Read the model definition and answer for the solid it produces. Units are mm, in the model's axes. Face numbers are marked on the shaded views. A direction names the side the tool comes from. Coordinates: 2 decimals unless noted, no trailing zeros. Loops run counter-clockwise (first coordinate to the right, second up) from the corner with the lowest first, then second, coordinate; pieces in that order, holes last. Notation, with made-up numbers: (9.25, -30.75) -> (23.25, -30.75) arc R15 ccw to (23.25, -5.75) -> close; hole circle Ø11 at (2, 54). An arc over 180 degrees is marked (long way). Answer in a Markdown table with one row per item.
```python
from build123d import *

# Parameters (mm, degrees)
BASE_EXTRUDE_DEPTH = 12.7
LPATTERN1_COUNT    = 2
LPATTERN1_PITCH    = 41.27246


with BuildPart() as part:
    # Sketch1 → Base-Extrude (new, symmetric)
    with BuildSketch(Plane.XY):
        with BuildLine():
            Line((-20.6375, 36.5125), (-20.6375, 2.6924))
            ThreePointArc((-20.6375, 2.6924), (-19.848914298, 0.788585702), (-17.9451, 0))
            Line((-17.9451, 0), (17.9451, 0))
            ThreePointArc((17.9451, 0), (19.848914298, 0.788585702), (20.6375, 2.6924))
            Line((20.6375, 2.6924), (20.6375, 36.5125))
            ThreePointArc((20.6375, 36.5125), (15.875, 41.275), (11.1125, 36.5125))
            Line((11.1125, 36.5125), (11.1125, 35.47745))
            ThreePointArc((11.1125, 35.47745), (12.4587, 34.13125), (13.8049, 35.47745))
            Line((13.8049, 35.47745), (13.8049, 36.5125))
            ThreePointArc((13.8049, 36.5125), (15.875, 38.5826), (17.9451, 36.5125))
            Line((17.9451, 36.5125), (17.9451, 2.6924))
            Line((17.9451, 2.6924), (-17.9451, 2.6924))
            Line((-17.9451, 2.6924), (-17.9451, 36.5125))
            ThreePointArc((-17.9451, 36.5125), (-15.875, 38.5826), (-13.8049, 36.5125))
            Line((-13.8049, 36.5125), (-13.8049, 35.47745))
            ThreePointArc((-13.8049, 35.47745), (-12.4587, 34.13125), (-11.1125, 35.47745))
            Line((-11.1125, 35.47745), (-11.1125, 36.5125))
            ThreePointArc((-11.1125, 36.5125), (-15.875, 41.275), (-20.6375, 36.5125))
        make_face()
    base_extrude = extrude(amount=BASE_EXTRUDE_DEPTH, both=True)

    # Mirror1: Base-Extrude across plane
    add(base_extrude.mirror(Plane.ZX))

    # LPattern1: Base-Extrude ×2
    with Locations(*[(0, i * LPATTERN1_PITCH, 0) for i in range(1, LPATTERN1_COUNT)]):
        add(base_extrude)


solid = part.part
```
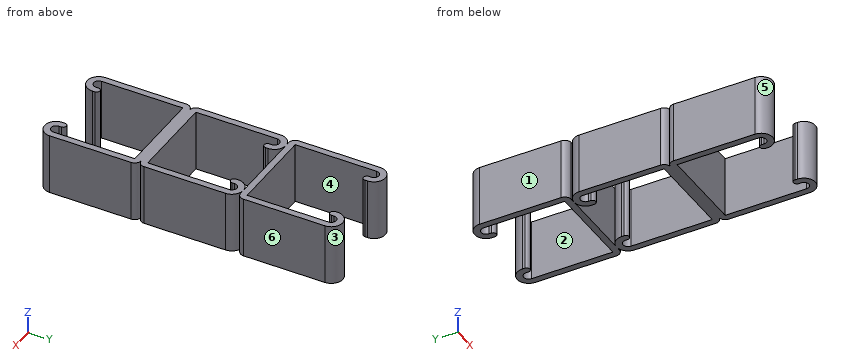
1. Find the intervals of material crossed by probe 1 along Y at (x, z) = (16, -9.25); probe 2 along X at (y, z) = (15, 10.5); probe 3 along Y at (x, z) = (1, -7.5), in increasing order.
A:
| item | result |
|---|---|
| probe 1 | y = -41.27 to -38.58, -2.69 to 2.69, 38.58 to 43.96, 79.85 to 82.55 |
| probe 2 | x = -20.64 to -17.95, 17.95 to 20.64 |
| probe 3 | y = -2.69 to 2.69, 41.27 to 43.96 |
2. The mould has two halves that part along Y. Classify the marked faces 3, 4, 5 and 6: pulls with the +Y half, pulls with the -Y half, needs draft (parallel to the pull), parting line crosses it, or undercut.
A:
| item | result |
|---|---|
| face 3 | pulls with the +Y half |
| face 4 | undercut |
| face 5 | pulls with the -Y half |
| face 6 | needs draft |
3. A tool of negligible diameter and unlimited length cuts with its end or side. For the marked faces 1 and 2, from which of +Z, -Z, +X, -X, +Y, -Y can it reach the whole face along a straight path? Write none if from no direction.
A:
| item | result |
|---|---|
| face 1 | +Z, -Z, -X, +Y, -Y |
| face 2 | +Z, -Z |
4. A cutting plane is placed at B-B on y = 52.5. Give the vertices of the cut face in (x, z).
A:
| item | result |
|---|---|
| outline | (-20.64, -12.7) -> (-17.95, -12.7) -> (-17.95, 12.7) -> (-20.64, 12.7) -> close; (17.95, -12.7) -> (20.64, -12.7) -> (20.64, 12.7) -> (17.95, 12.7) -> close |
5. A cutting plane is placed at A-A on x = 10. Give the vertices of the cut face in (y, z), and give its area (3 significant figures).
A:
| item | result |
|---|---|
| outline | (-2.69, -12.7) -> (2.69, -12.7) -> (2.69, 12.7) -> (-2.69, 12.7) -> close; (41.27, -12.7) -> (43.96, -12.7) -> (43.96, 12.7) -> (41.27, 12.7) -> close |
| area | 205 mm2 |
6. Given pin 1 Ø1 at (x, z) = (-16.5, -1) entering from -Y; pin 2 Ø3 at (x, z) = (-13.5, 4.5) entering from +Y; pin 3 Ø1.5 at (x, z) = (8.5, -9.5) entering from +Y, each flat-ended and moving along its own axis, determine where each tip first touches the part or whether it passes through.
A:
| item | result |
|---|---|
| pin 1 | stops at y = -41.27 |
| pin 2 | stops at y = 82.47 |
| pin 3 | stops at y = 43.96 |
